from build123d import *

# Parameters (mm, degrees)
F0_W          = 20
F0_H          = 60
F1_DEPTH      = 20
F1_DEPTH_BACK = 20
F2_SIZE       = 0.2
F3_R          = 6
F4_DEPTH      = 17
F4_DEPTH_BACK = 17
F5_R          = 0.2
F6_SIZE       = 0.2
F8_W          = 1
F8_H          = 0.65


with BuildPart() as f1:
    # F0 (on Front) → F1 (new body, two sides)
    with BuildSketch(Plane.XZ) as f1_sk:
        Rectangle(F0_W, F0_H)
    extrude(amount=F1_DEPTH)
    extrude(f1_sk.sketch, amount=-F1_DEPTH_BACK)

    # F2
    f2_edges = [f1.edges().sort_by_distance(p)[0] for p in [
        (10, 0, 30),
        (-10, 0, -30),
        (10, 0, -30),
        (-10, 0, 30),
        (0, 20, 30),
        (0, -20, 30),
        (0, 20, -30),
        (0, -20, -30),
        (-10, 20, 0),
        (-10, -20, 0),
        (10, 20, 0),
        (10, -20, 0),
    ]]
    chamfer(f2_edges, length=F2_SIZE)

    # F3 (on Right) → F4 (join, two sides)
    with BuildSketch(Plane.YZ) as f4_sk:
        with Locations((0, 15)):
            Circle(F3_R)
    extrude(amount=-F4_DEPTH)
    extrude(f4_sk.sketch, amount=F4_DEPTH_BACK)

    # F5
    f5_edges = [f1.edges().sort_by_distance(p)[0] for p in [
        (-10, -6, 15),
        (10, -6, 15),
    ]]
    fillet(f5_edges, radius=F5_R)

    # F6
    f6_edges = [f1.edges().sort_by_distance(p)[0] for p in [
        (17, -6, 15),
        (-17, -6, 15),
    ]]
    chamfer(f6_edges, length=F6_SIZE)

    # F8 (on offset) → F9 (revolve, cut)
    with BuildSketch(Plane.XY.offset(15)):
        with Locations((-15.7, 5.675)):
            Rectangle(F8_W, F8_H)
        with Locations((15.7, 5.675)):
            Rectangle(F8_W, F8_H)
    revolve(axis=Axis((0.9265579283, 0, 15), (1, 0, 0)), mode=Mode.SUBTRACT)


solid = f1.part
Source: CAD feature listing. Evaluate the final solid. Frame: model axes, mm. A direction names the side the tool comes from. Give positions to 0.01 mm unless a question says otherwise; leave off trailing zeros. Loops run counter-clockwise (first coordinate to the right, second up) from the corner with the lowest first, then second, coordinate; pieces in that order, holes last. Notation, with made-up numbers: (65, 38.25) -> (121, 38.25) arc R12 ccw to (121, 43.25) -> close; hole circle Ø9 at (23, -11.5). An arc over 180 degrees is marked (long way). Use a Markdown table: item, result. Add a question column.
1) Section query C-C, the plane x = 12.5. Return the cut outline in (y, z).
2) Section query A-A, the plane z = -6.5. Return the cut outline in (x, y), then the cut area to 3 significant figures.
3) Reachability of faces 1 (the face through (-13, -6, 15)), 2 (the face through (13, -6, 15)), 3 (the face through (15.71, 2.88, 19.51)) from +Z, -Z, +X, -X, +Y, -Y: full face, straight path, thin tool, end or side. Return the list, or none.
4) Line query: line 1 along X through (y, z) = (2.5, -13.5); line 2 along Y through (x, z) = (14.5, 10.5). Output: solid intervals per line, ascending. Write a range as [from, to].
5) Section query B-B, the plane y = 7.5. Return the cut outline in (x, z).
6) Pull-direction query (Y, two-part tool) for faces 4 (the face through (0, 20, 0)), 5 (the face through (-15.69, 2.88, 19.51)), 6 (the face through (0, 0, -30)); classes: +Y half, -Y half, draft (parallel to the pull), parting line (faces both ways), or undercut.
7) First-contact query: pin 1 (3 mm diameter, centred on y = 11, z = -2.5, fed in from -X); pin 2 (5 mm diameter, centred on x = 10, y = -1, fed in from -Z); pin 3 (1.5 mm diameter, centred on x = 12.5, y = 14.5, fed in from +Z). Flat tips, straight axial feed; report the tip coordinate or a pass-through.
Numbers:
| question | item | result |
|---|---|---|
| 1 | outline | circle Ø12 at (0, 15) |
| 2 | outline | (-10, -19.8) -> (-9.8, -20) -> (9.8, -20) -> (10, -19.8) -> (10, 19.8) -> (9.8, 20) -> (-9.8, 20) -> (-10, 19.8) -> close |
| 2 | area | 800 mm2 |
| 3 | face 1 | -X |
| 3 | face 2 | +X |
| 3 | face 3 | none |
| 4 | line 1 | x = [-10, 10] |
| 4 | line 2 | y = [-3.97, 3.97] |
| 5 | outline | (-10, -29.8) -> (-9.8, -30) -> (9.8, -30) -> (10, -29.8) -> (10, 29.8) -> (9.8, 30) -> (-9.8, 30) -> (-10, 29.8) -> close |
| 6 | face 4 | +Y half |
| 6 | face 5 | parting line |
| 6 | face 6 | draft |
| 7 | pin 1 | stops at x = -10 |
| 7 | pin 2 | stops at z = -30 |
| 7 | pin 3 | passes through |
